Part model, mm, in its own coordinate system. Face numbers are marked on the shaded views. A direction names the side the tool comes from. Round coordinates to 2 decimals unless told otherwise and drop trailing zeros. Write each loop counter-clockwise with the first axis right and the second up, starting at its lowest first coordinate (ties: lowest second). Pieces come first, ordered by that corner, then holes. Notation, with made-up numbers: (-10, 33.5) -> (17, 33.5) arc R14 ccw to (17, 43.5) -> close; hole circle Ø9 at (-38, -23.75). An arc over 180 degrees is marked (long way). Return JSON: item names as keys, results as strings. Group by question number.
(1) Saw through at B-B (y = -7). State how many separate pieces and enclosed holes the cut face has, plus the area to 3 significant figures.
(2) Tool access for the marked faces 1, 2 and 3: list every direction of +Z, -Z, +X, -X, +Y, -Y with a clear straight run to the whole face (end or side of a thin tool).
(3) Drill centre lines: L1, parallel to X at y = -10, z = 26.5; L2, parallel to X at y = -25, z = 3.5 (3 decimals); L3, parallel to Z at x = -17, y = 5. Where is each one in solid material? Low to high. Write a range as from..to.
(4) Drop flat-ended pins along their axis: pin 1 Ø4 at (x, y) = (6.35, 26.99) entering from +Z; pin 2 Ø5 at (x, y) = (-21.5, 16.5) entering from +Z; pin 3 Ø1.4 at (x, z) = (18.5, 2.5) entering from +Y; pin 4 Ø6 at (x, y) = (25.5, 2) entering from +Z. Give the stop position or say it passes through.
(5) Saw through at C-C (z = 15.5). List the corners of the cut face in (x, y), plus the area to 3 significant figures.
(6) Saw through at A-A (x = -19.05). List the corners of the cut face in (y, z), plus the area to 3 significant figures.
(7) Saw through at D-D (x = -31.75). List the corners of the cut face in (y, z), plus the area to 3 significant figures.
(8) Mould opens along Y. For the marked faces 4, 5 and 6 say: +Y half, -Y half, draft (parallel to the pull), parting line (faces both ways), or undercut.
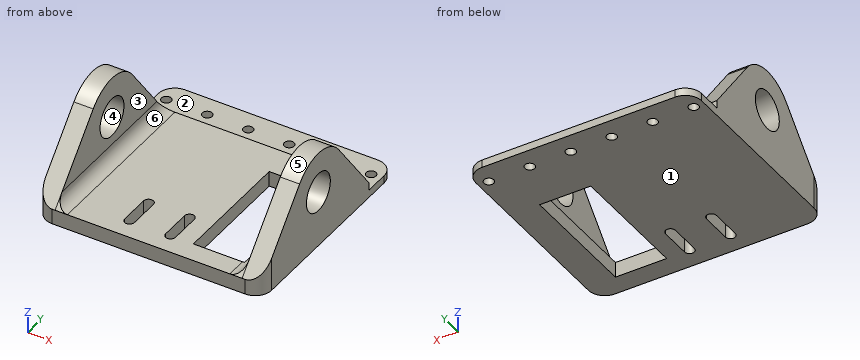
from build123d import *

# Parameters (mm, degrees)
F0_W          = 70
F0_H          = 66.675
F1_DEPTH      = 4.7625
F2_R          = 6
F3_DEPTH      = 70
F4_W          = 58
F4_H          = 53.975
F5_DEPTH      = 25.401
F6_W          = 15.875
F6_H          = 38.1
F7_DEPTH      = 4.7625
F9_DEPTH      = 25.4
F10_W         = 70
F10_H         = 12.7
F11_DEPTH     = 2.38125
F12_R         = 1.524
F13_DEPTH     = 2.38125
F14_R         = 5.08
F15_T4_DEPTH  = 53.975
F15_T10_DEPTH = 53.975
F15_T17_DEPTH = 53.975
F15_T24_DEPTH = 53.975
F15_T31_DEPTH = 53.975
F15_T38_DEPTH = 53.975
F16_R         = 5.08


# Not quite as in the source:
# - a fillet or chamfer that OpenCascade refuses, or shapes differently, is made with other operations: its cross-section is extruded or revolved along the edge and cut away or added
# - a feature of the source that left no trace in its solid (it failed there, or was rolled back) is left out


with BuildPart() as f1:
    # F0 (on Top) → F1 (new body)
    with BuildSketch(Plane.XY):
        Rectangle(F0_W, F0_H)
    extrude(amount=F1_DEPTH)

    # F2 (on face) → F3 (join, through all)
    with BuildSketch(Plane(origin=(-35, 0, 0), x_dir=(0, -1, 0), z_dir=(-1, 0, 0))):
        with BuildLine():
            ThreePointArc((-5.3975, 25.0825), (-7.2857778852, 21.4785926284), (-7.9375, 17.4625))
            Line((-7.9375, 17.4625), (-7.9375, 4.7625))
            Line((-7.9375, 4.7625), (17.4625, 4.7625))
            Line((17.4625, 4.7625), (17.4625, 17.4625))
            ThreePointArc((17.4625, 17.4625), (16.6159891988, 22.0215343072), (14.1893041237, 25.9728092784))
            ThreePointArc((14.1893041237, 25.9728092784), (4.1858227063, 30.1494004607), (-5.3975, 25.0825))
        make_face()
        with Locations((4.7625, 17.4625)):
            Circle(F2_R, mode=Mode.SUBTRACT)
        with BuildLine():
            Line((-7.9375, 4.7625), (-7.9375, 17.4625))
            ThreePointArc((-7.9375, 17.4625), (-7.2857778852, 21.4785926284), (-5.3975, 25.0825))
            Line((-5.3975, 25.0825), (-20.6375, 4.7625))
            Line((-20.6375, 4.7625), (-7.9375, 4.7625))
        make_face()
        with BuildLine():
            Line((17.4625, 17.4625), (17.4625, 4.7625))
            Line((17.4625, 4.7625), (33.3375, 4.7625))
            Line((33.3375, 4.7625), (14.1893041237, 25.9728092784))
            ThreePointArc((14.1893041237, 25.9728092784), (16.6159891988, 22.0215343072), (17.4625, 17.4625))
        make_face()
    extrude(amount=-F3_DEPTH)

    # F4 (on face) → F5 (cut, through all)
    with BuildSketch(Plane.XY.offset(4.7625)):
        with Locations((0, -6.35)):
            Rectangle(F4_W, F4_H)
    extrude(amount=F5_DEPTH, mode=Mode.SUBTRACT)

    # F6 (on face) → F7 (cut, through all)
    with BuildSketch(Plane.XY.offset(4.7625)):
        with Locations((17.8875, -7.9375)):
            Rectangle(F6_W, F6_H)
    extrude(amount=-F7_DEPTH, mode=Mode.SUBTRACT)

    # F8 (on face) → F9 (cut)
    with BuildSketch(Plane(origin=(0, 0, 0), x_dir=(1, 0, 0), z_dir=(0, 0, -1))):
        with BuildLine():
            Line((1.345, 26.9875), (1.345, 17.4625))
            ThreePointArc((1.345, 17.4625), (2.869, 15.9385), (4.393, 17.4625))
            Line((4.393, 17.4625), (4.393, 26.9875))
            ThreePointArc((4.393, 26.9875), (2.869, 28.5115), (1.345, 26.9875))
        make_face()
        with BuildLine():
            Line((-11.355, 26.9875), (-11.355, 17.4625))
            ThreePointArc((-11.355, 17.4625), (-9.831, 15.9385), (-8.307, 17.4625))
            Line((-8.307, 17.4625), (-8.307, 26.9875))
            ThreePointArc((-8.307, 26.9875), (-9.831, 28.5115), (-11.355, 26.9875))
        make_face()
    extrude(amount=-F9_DEPTH, mode=Mode.SUBTRACT)

    # F10 (on face) → F11 (cut)
    with BuildSketch(Plane.XY.offset(4.7625)):
        with Locations((0, 26.9875)):
            Rectangle(F10_W, F10_H)
    extrude(amount=-F11_DEPTH, mode=Mode.SUBTRACT)

    # F12 (on face) → F13 (cut, through all)
    with BuildSketch(Plane.XY.offset(2.38125)):
        with Locations((-31.75, 26.9875)):
            Circle(F12_R)
        with Locations((-19.05, 26.9875)):
            Circle(F12_R)
        with Locations((-6.35, 26.9875)):
            Circle(F12_R)
        with Locations((6.35, 26.9875)):
            Circle(F12_R)
        with Locations((19.05, 26.9875)):
            Circle(F12_R)
        with Locations((31.75, 26.9875)):
            Circle(F12_R)
    extrude(amount=-F13_DEPTH, mode=Mode.SUBTRACT)

    # F14
    f14_edges = [f1.edges().sort_by_distance(p)[0] for p in [
        (-35, 33.3375, 1.190625),
        (35, 33.3375, 1.190625),
    ]]
    fillet(f14_edges, radius=F14_R)

    # F15: fillet of radius 3.81 on 2 edges, made by hand


with BuildPart() as f15_tool2:
    # F15_s3 → F15_t4 (new body)
    with BuildSketch(Plane.XZ.offset(-20.6375)):
        with BuildLine():
            ThreePointArc((-25.19, 4.7625), (-27.8840768363, 5.8784231637), (-29, 8.5725))
            Line((-29, 8.5725), (-29, 4.7625))
            Line((-29, 4.7625), (-25.19, 4.7625))
        make_face()
    extrude(amount=F15_T4_DEPTH)

    split(bisect_by=Plane(origin=(0, -20.7365394835, 18.7204870337), x_dir=(1, 0, 0), z_dir=(0, 0.7422680412, -0.6701030928)), keep=Keep.TOP)

    split(bisect_by=Plane(origin=(0, 15.494, 11.6205), x_dir=(1, 0, 0), z_dir=(0, -0.8, -0.6)), keep=Keep.TOP)


with BuildPart() as f1_1:
    add(f1.part)

    # F15_t1: union F15_tool2
    add(f15_tool2.part)


with BuildPart() as f15_tool8:
    # F15_s9 → F15_t10 (new body)
    with BuildSketch(Plane.XZ.offset(33.3375)):
        with BuildLine():
            ThreePointArc((25.19, 4.7625), (27.8840768363, 5.8784231637), (29, 8.5725))
            Line((29, 8.5725), (29, 4.7625))
            Line((29, 4.7625), (25.19, 4.7625))
        make_face()
    extrude(amount=-F15_T10_DEPTH)

    split(bisect_by=Plane(origin=(0, -20.7365394835, 18.7204870337), x_dir=(1, 0, 0), z_dir=(0, 0.7422680412, -0.6701030928)), keep=Keep.TOP)

    split(bisect_by=Plane.XZ.offset(26.9875), keep=Keep.TOP)

    split(bisect_by=Plane.YZ.offset(25.825), keep=Keep.BOTTOM)


with BuildPart() as f1_2:
    add(f1_1.part)

    # F15_t7: union F15_tool8
    add(f15_tool8.part)


with BuildPart() as f15_tool15:
    # F15_s16 → F15_t17 (new body)
    with BuildSketch(Plane.XZ.offset(33.3375)):
        with BuildLine():
            ThreePointArc((25.19, 4.7625), (27.8840768363, 5.8784231637), (29, 8.5725))
            Line((29, 8.5725), (29, 4.7625))
            Line((29, 4.7625), (25.19, 4.7625))
        make_face()
    extrude(amount=-F15_T17_DEPTH)

    split(bisect_by=Plane(origin=(0, -20.7365394835, 18.7204870337), x_dir=(1, 0, 0), z_dir=(0, 0.7422680412, -0.6701030928)), keep=Keep.TOP)

    split(bisect_by=Plane.XZ.offset(26.9875), keep=Keep.TOP)

    split(bisect_by=Plane.YZ.offset(25.825), keep=Keep.TOP)


with BuildPart() as f1_3:
    add(f1_2.part)

    # F15_t14: union F15_tool15
    add(f15_tool15.part)


with BuildPart() as f15_tool22:
    # F15_s23 → F15_t24 (new body)
    with BuildSketch(Plane.XZ.offset(33.3375)):
        with BuildLine():
            ThreePointArc((25.19, 4.7625), (27.8840768363, 5.8784231637), (29, 8.5725))
            Line((29, 8.5725), (29, 4.7625))
            Line((29, 4.7625), (25.19, 4.7625))
        make_face()
    extrude(amount=-F15_T24_DEPTH)

    split(bisect_by=Plane.XZ.offset(26.9875), keep=Keep.BOTTOM)

    split(bisect_by=Plane.YZ.offset(25.825), keep=Keep.TOP)

    split(bisect_by=Plane.XZ.offset(-11.1125), keep=Keep.TOP)


with BuildPart() as f1_4:
    add(f1_3.part)

    # F15_t21: union F15_tool22
    add(f15_tool22.part)


with BuildPart() as f15_tool29:
    # F15_s30 → F15_t31 (new body)
    with BuildSketch(Plane.XZ.offset(33.3375)):
        with BuildLine():
            ThreePointArc((25.19, 4.7625), (27.8840768363, 5.8784231637), (29, 8.5725))
            Line((29, 8.5725), (29, 4.7625))
            Line((29, 4.7625), (25.19, 4.7625))
        make_face()
    extrude(amount=-F15_T31_DEPTH)

    split(bisect_by=Plane(origin=(0, 15.494, 11.6205), x_dir=(1, 0, 0), z_dir=(0, -0.8, -0.6)), keep=Keep.TOP)

    split(bisect_by=Plane.YZ.offset(25.825), keep=Keep.BOTTOM)

    split(bisect_by=Plane.XZ.offset(-11.1125), keep=Keep.BOTTOM)


with BuildPart() as f1_5:
    add(f1_4.part)

    # F15_t28: union F15_tool29
    add(f15_tool29.part)


with BuildPart() as f15_tool36:
    # F15_s37 → F15_t38 (new body)
    with BuildSketch(Plane.XZ.offset(33.3375)):
        with BuildLine():
            ThreePointArc((25.19, 4.7625), (27.8840768363, 5.8784231637), (29, 8.5725))
            Line((29, 8.5725), (29, 4.7625))
            Line((29, 4.7625), (25.19, 4.7625))
        make_face()
    extrude(amount=-F15_T38_DEPTH)

    split(bisect_by=Plane(origin=(0, 15.494, 11.6205), x_dir=(1, 0, 0), z_dir=(0, -0.8, -0.6)), keep=Keep.TOP)

    split(bisect_by=Plane.YZ.offset(25.825), keep=Keep.TOP)

    split(bisect_by=Plane.XZ.offset(-11.1125), keep=Keep.BOTTOM)


with BuildPart() as f1_6:
    add(f1_5.part)

    # F15_t35: union F15_tool36
    add(f15_tool36.part)

    # F16
    f16_edges = [f1_6.edges().sort_by_distance(p)[0] for p in [
        (35, -33.3375, 2.38125),
        (-35, -33.3375, 2.38125),
    ]]
    fillet(f16_edges, radius=F16_R)


solid = f1_6.part
Computed values:
{
 "1": {"separate pieces": "4", "enclosed holes": "0", "area": "433 mm2"},
 "2": {"face 1": "-Z, +X, -X, +Y, -Y", "face 2": "+Z, +X, -X, +Y", "face 3": "+Z, +Y, -Y"},
 "3": {"L1": "-35..-29, 29..35", "L2": "-35..-11.355, -8.307..1.345, 4.393..9.95, 25.825..35", "L3": "0..4.76"},
 "4": {"pin 1": "z = 2.38", "pin 2": "z = 4.76", "pin 3": "y = 33.34", "pin 4": "z = 6.69"},
 "5": {"outline": "(-35, -23.64) -> (-29, -23.64) -> (-29, -10.43) -> (-35, -10.43) -> close; (-35, 0.91) -> (-29, 0.91) -> (-29, 12.58) -> (-35, 12.58) -> close; (29, -23.64) -> (35, -23.64) -> (35, -10.43) -> (29, -10.43) -> close; (29, 0.91) -> (35, 0.91) -> (35, 12.58) -> (29, 12.58) -> close", "area": "299 mm2"},
 "6": {"outline": "(-33.34, 0) -> (25.46, 0) -> (25.46, 2.38) -> (20.64, 2.38) -> (20.64, 4.76) -> (-33.34, 4.76) -> close; (28.51, 0) -> (33.34, 0) -> (33.34, 2.38) -> (28.51, 2.38) -> close", "area": "280 mm2"},
 "7": {"outline": "(-33, 0) -> (25.46, 0) -> (25.46, 2.38) -> (20.64, 2.38) -> (20.64, 4.76) -> (5.4, 25.08) arc R12.7 ccw to (-14.19, 25.97) -> (-33, 5.14) -> close; (28.51, 0) -> (33, 0) -> (33, 2.38) -> (28.51, 2.38) -> close; hole circle Ø12 at (-4.76, 17.46)", "area": "992 mm2"},
 "8": {"face 4": "undercut", "face 5": "parting line", "face 6": "draft"}
}
